from build123d import *

# Parameters (mm, degrees)
SKETCH2_W                                         = 215
SKETCH2_H                                         = 30
BOSS_EXTRUDE1_DEPTH                               = 3.5
SKETCH4_W                                         = 30
SKETCH4_H                                         = 8
SKETCH4_W_2                                       = 25
BOSS_EXTRUDE2_DEPTH                               = 28
CBORE_FOR_M6_HEX_HEAD_BOLT1_D                     = 14
CBORE_FOR_M6_HEX_HEAD_BOLT1_CBORE_D               = 16
CBORE_FOR_M6_HEX_HEAD_BOLT1_CBORE_DEPTH           = 6
CBORE_FOR_M6_HEX_HEAD_BOLT1_ON_FACE_2_D           = 14
CBORE_FOR_M6_HEX_HEAD_BOLT1_ON_FACE_2_CBORE_D     = 16
CBORE_FOR_M6_HEX_HEAD_BOLT1_ON_FACE_2_CBORE_DEPTH = 6
FILLET1_R                                         = 10
HOLES_TBD_R                                       = 1.65
CUT_EXTRUDE1_DEPTH                                = 113.094825929
FILLET2_R                                         = 3


with BuildPart() as part:
    # Sketch2 → Boss-Extrude1 (new body)
    with BuildSketch(Plane(origin=(0, 0, 0), x_dir=(1, 0, 0), z_dir=(0, 1, 0))):
        Rectangle(SKETCH2_W, SKETCH2_H)
    extrude(amount=BOSS_EXTRUDE1_DEPTH)

    # Sketch4 → Boss-Extrude2 (add)
    with BuildSketch(Plane(origin=(0, 3.5, 0), x_dir=(1, 0, 0), z_dir=(0, 1, 0))):
        with Locations((0, -11)):
            Rectangle(SKETCH4_W, SKETCH4_H)
        with Locations((95, 11)):
            Rectangle(SKETCH4_W_2, SKETCH4_H)
        with Locations((0, 11)):
            Rectangle(SKETCH4_W, SKETCH4_H)
    extrude(amount=BOSS_EXTRUDE2_DEPTH)

    # CBORE for M6 Hex Head Bolt1 (through all)
    with Locations(Plane(origin=(0, 17.5, 15), x_dir=(1, 0, 0), z_dir=(0, 0, 1))):
        with Locations((0, 0)):
            CounterBoreHole(CBORE_FOR_M6_HEX_HEAD_BOLT1_D / 2, CBORE_FOR_M6_HEX_HEAD_BOLT1_CBORE_D / 2, CBORE_FOR_M6_HEX_HEAD_BOLT1_CBORE_DEPTH)

    # CBORE for M6 Hex Head Bolt1 on face 2 (through all)
    with Locations(Plane(origin=(0, 17.5, -15), x_dir=(-1, 0, 0), z_dir=(0, 0, -1))):
        with Locations((0, 0), (-95, 0)):
            CounterBoreHole(CBORE_FOR_M6_HEX_HEAD_BOLT1_ON_FACE_2_D / 2, CBORE_FOR_M6_HEX_HEAD_BOLT1_ON_FACE_2_CBORE_D / 2, CBORE_FOR_M6_HEX_HEAD_BOLT1_ON_FACE_2_CBORE_DEPTH)

    # Fillet1
    fillet1_edges = [part.edges().sort_by_distance(p)[0] for p in [
        (107.5, 31.5, -11),
        (82.5, 31.5, -11),
        (-15, 31.5, 11),
        (15, 31.5, 11),
        (-15, 31.5, -11),
        (15, 31.5, -11),
    ]]
    fillet(fillet1_edges, radius=FILLET1_R)

    # HOLES TBD → Cut-Extrude1 (cut, through all)
    with BuildSketch(Plane(origin=(0, 3.5, 0), x_dir=(1, 0, 0), z_dir=(0, 1, 0))):
        with Locations(Location((-100, 0, 0), (0, 0, 270))):
            Circle(HOLES_TBD_R)
        with Locations(Location((100, 0, 0), (0, 0, 270))):
            Circle(HOLES_TBD_R)
    extrude(amount=-CUT_EXTRUDE1_DEPTH, mode=Mode.SUBTRACT)

    # Fillet2
    fillet2_edges = [part.edges().sort_by_distance(p)[0] for p in [
        (82.5, 3.5, -11),
        (95, 3.5, -7),
        (-15, 3.5, 11),
        (15, 3.5, 11),
        (0, 3.5, 7),
        (-15, 3.5, -11),
        (0, 3.5, -7),
        (15, 3.5, -11),
    ]]
    fillet(fillet2_edges, radius=FILLET2_R)


solid = part.part
CAD build for the part. Positions are in the model's coordinates, mm. A direction names the side the tool comes from. Coordinates: 2 decimals unless noted, no trailing zeros. Write each loop counter-clockwise with the first axis right and the second up, starting at its lowest first coordinate (ties: lowest second). Pieces come first, ordered by that corner, then holes. Notation, with made-up numbers: M 58,32 L 88,32 A20 cw 88,58 Z; hole C -38,76.5 d11. An arc over 180 degrees is marked long. Answer as a JSON object with one key per item and string values. Group by question number.
1) Saw through at D-D (y = 19.5). Give the number of separate pieces and of enclosed holes in the cut face, plus the area to 3 significant figures.
2) Saw through at A-A (x = 0). Write the cut outline in (y, z).
3) Wall check: line 1 (X direction, y = 1.4, z = 0); line 2 (Z direction, x = 10, y = 28.5). Give the ranges that are in metal, low to high. Write a range as from..to.
4) Tool access for faces 4 (the face through (15, 14, -11)), 5 (the face through (-7, 19, 7)), 6 (the face through (102.992, 17.852, -12.042)): list every direction of +Z, -Z, +X, -X, +Y, -Y with a clear straight run to the whole face (end or side of a thin tool).
5) Saw through at C-C (y = 29). Write the cut outline in (x, z), plus the area to 3 significant figures.
6) Pin check, flat tips, straight feed: pin 1 Ø4 at (y, z) = (13, 11.5) entering from +X; pin 2 Ø12.5 at (x, y) = (98, 17) entering from +Z; pin 3 Ø17.5 at (x, y) = (-2.5, 17) entering from +Z; pin 4 Ø10 at (x, y) = (25, 13) entering from -Z. Stop position of each tip, or through.
7) Mould opens along X. For faces 1 (the face through (-15, 14, -11)), 2 (the face through (0, 31.5, -11)), 3 (the face through (95, 10, -9)) say: +X half, -X half, draft (parallel to the pull), parting line (faces both ways), or undercut.
8) Saw through at B-B (x = 95). Write the cut outline in (y, z).
Values follow:
{
 "1": {"separate pieces": "6", "enclosed holes": "0", "area": "321 mm2"},
 "2": {"outline": "M 0,-15 L 9.5,-15 L 9.5,-9 L 10.5,-9 L 10.5,-7 L 6.5,-7 A3 cw 3.5,-4 L 3.5,4 A3 cw 6.5,7 L 10.5,7 L 10.5,9 L 9.5,9 L 9.5,15 L 0,15 Z; M 24.5,-9 L 25.5,-9 L 25.5,-15 L 31.5,-15 L 31.5,-7 L 24.5,-7 Z; M 24.5,7 L 31.5,7 L 31.5,15 L 25.5,15 L 25.5,9 L 24.5,9 Z"},
 "3": {"line 1": "x = -107.5..-101.65, -98.35..98.35, 101.65..107.5", "line 2": "z = -15..-7, 7..15"},
 "4": {"face 4": "+Z, -Z, +Y", "face 5": "+X, -X, +Y", "face 6": "-Z"},
 "5": {"outline": "M -11.61,-15 L 11.61,-15 L 11.61,-7 L -11.61,-7 Z; M -11.61,7 L 11.61,7 L 11.61,15 L -11.61,15 Z; M 85.89,-15 L 104.11,-15 L 104.11,-7 L 85.89,-7 Z", "area": "517 mm2"},
 "6": {"pin 1": "stops at x = 15", "pin 2": "stops at z = -7", "pin 3": "stops at z = 15", "pin 4": "passes through"},
 "7": {"face 1": "-X half", "face 2": "draft", "face 3": "undercut"},
 "8": {"outline": "M 0,-15 L 9.5,-15 L 9.5,-9 L 10.5,-9 L 10.5,-7 L 6.5,-7 A3 cw 3.5,-4 L 3.5,15 L 0,15 Z; M 24.5,-9 L 25.5,-9 L 25.5,-15 L 31.5,-15 L 31.5,-7 L 24.5,-7 Z"}
}
